```python
from build123d import *

# Parameters (mm, degrees)
SKETCH1_R           = 2.5
BOSS_EXTRUDE1_DEPTH = 370


with BuildPart() as part:
    # Sketch1 → Boss-Extrude1 (new body)
    with BuildSketch(Plane(origin=(0, 0, 0), x_dir=(1, 0, 0), z_dir=(0, 1, 0))):
        with BuildLine():
            Line((-10, 4.65), (-9.8, 4.65))
            Line((-9.8, 4.65), (-9.8, 4.4))
            ThreePointArc((-9.8, 4.4), (-9.741421356, 4.258578644), (-9.6, 4.2))
            Line((-9.6, 4.2), (-8.4, 4.2))
            ThreePointArc((-8.4, 4.2), (-8.258578644, 4.258578644), (-8.2, 4.4))
            Line((-8.2, 4.4), (-8.2, 5.45))
            ThreePointArc((-8.2, 5.45), (-8.141421356, 5.591421356), (-8, 5.65))
            Line((-8, 5.65), (-6.832842712, 5.65))
            ThreePointArc((-6.832842712, 5.65), (-6.756306026, 5.634775907), (-6.691421356, 5.591421356))
            Line((-6.691421356, 5.591421356), (-4.058578644, 2.958578644))
            ThreePointArc((-4.058578644, 2.958578644), (-4.015224093, 2.893693974), (-4, 2.817157288))
            Line((-4, 2.817157288), (-4, -2.817157288))
            ThreePointArc((-4, -2.817157288), (-4.015224093, -2.893693974), (-4.058578644, -2.958578644))
            Line((-4.058578644, -2.958578644), (-6.691421356, -5.591421356))
            ThreePointArc((-6.691421356, -5.591421356), (-6.756306026, -5.634775907), (-6.832842712, -5.65))
            Line((-6.832842712, -5.65), (-8, -5.65))
            ThreePointArc((-8, -5.65), (-8.141421356, -5.591421356), (-8.2, -5.45))
            Line((-8.2, -5.45), (-8.2, -4.4))
            ThreePointArc((-8.2, -4.4), (-8.258578644, -4.258578644), (-8.4, -4.2))
            Line((-8.4, -4.2), (-9.6, -4.2))
            ThreePointArc((-9.6, -4.2), (-9.741421356, -4.258578644), (-9.8, -4.4))
            Line((-9.8, -4.4), (-9.8, -4.65))
            Line((-9.8, -4.65), (-10, -4.65))
            Line((-10, -4.65), (-10, -9.8))
            ThreePointArc((-10, -9.8), (-9.941421356, -9.941421356), (-9.8, -10))
            Line((-9.8, -10), (-4.65, -10))
            Line((-4.65, -10), (-4.65, -9.8))
            Line((-4.65, -9.8), (-4.4, -9.8))
            ThreePointArc((-4.4, -9.8), (-4.258578644, -9.741421356), (-4.2, -9.6))
            Line((-4.2, -9.6), (-4.2, -8.4))
            ThreePointArc((-4.2, -8.4), (-4.258578644, -8.258578644), (-4.4, -8.2))
            Line((-4.4, -8.2), (-5.45, -8.2))
            ThreePointArc((-5.45, -8.2), (-5.591421356, -8.141421356), (-5.65, -8))
            Line((-5.65, -8), (-5.65, -6.832842712))
            ThreePointArc((-5.65, -6.832842712), (-5.634775907, -6.756306026), (-5.591421356, -6.691421356))
            Line((-5.591421356, -6.691421356), (-2.958578644, -4.058578644))
            ThreePointArc((-2.958578644, -4.058578644), (-2.893693974, -4.015224093), (-2.817157288, -4))
            Line((-2.817157288, -4), (2.817157288, -4))
            ThreePointArc((2.817157288, -4), (2.893693974, -4.015224093), (2.958578644, -4.058578644))
            Line((2.958578644, -4.058578644), (5.591421356, -6.691421356))
            ThreePointArc((5.591421356, -6.691421356), (5.634775907, -6.756306026), (5.65, -6.832842712))
            Line((5.65, -6.832842712), (5.65, -8))
            ThreePointArc((5.65, -8), (5.591421356, -8.141421356), (5.45, -8.2))
            Line((5.45, -8.2), (4.4, -8.2))
            ThreePointArc((4.4, -8.2), (4.258578644, -8.258578644), (4.2, -8.4))
            Line((4.2, -8.4), (4.2, -9.6))
            ThreePointArc((4.2, -9.6), (4.258578644, -9.741421356), (4.4, -9.8))
            Line((4.4, -9.8), (4.65, -9.8))
            Line((4.65, -9.8), (4.65, -10))
            Line((4.65, -10), (9.8, -10))
            ThreePointArc((9.8, -10), (9.941421356, -9.941421356), (10, -9.8))
            Line((10, -9.8), (10, -4.65))
            Line((10, -4.65), (9.8, -4.65))
            Line((9.8, -4.65), (9.8, -4.4))
            ThreePointArc((9.8, -4.4), (9.741421356, -4.258578644), (9.6, -4.2))
            Line((9.6, -4.2), (8.4, -4.2))
            ThreePointArc((8.4, -4.2), (8.258578644, -4.258578644), (8.2, -4.4))
            Line((8.2, -4.4), (8.2, -5.45))
            ThreePointArc((8.2, -5.45), (8.141421356, -5.591421356), (8, -5.65))
            Line((8, -5.65), (6.832842712, -5.65))
            ThreePointArc((6.832842712, -5.65), (6.756306026, -5.634775907), (6.691421356, -5.591421356))
            Line((6.691421356, -5.591421356), (4.058578644, -2.958578644))
            ThreePointArc((4.058578644, -2.958578644), (4.015224093, -2.893693974), (4, -2.817157288))
            Line((4, -2.817157288), (4, 2.817157288))
            ThreePointArc((4, 2.817157288), (4.015224093, 2.893693974), (4.058578644, 2.958578644))
            Line((4.058578644, 2.958578644), (6.691421356, 5.591421356))
            ThreePointArc((6.691421356, 5.591421356), (6.756306026, 5.634775907), (6.832842712, 5.65))
            Line((6.832842712, 5.65), (8, 5.65))
            ThreePointArc((8, 5.65), (8.141421356, 5.591421356), (8.2, 5.45))
            Line((8.2, 5.45), (8.2, 4.4))
            ThreePointArc((8.2, 4.4), (8.258578644, 4.258578644), (8.4, 4.2))
            Line((8.4, 4.2), (9.6, 4.2))
            ThreePointArc((9.6, 4.2), (9.741421356, 4.258578644), (9.8, 4.4))
            Line((9.8, 4.4), (9.8, 4.65))
            Line((9.8, 4.65), (10, 4.65))
            Line((10, 4.65), (10, 9.8))
            ThreePointArc((10, 9.8), (9.941421356, 9.941421356), (9.8, 10))
            Line((9.8, 10), (4.65, 10))
            Line((4.65, 10), (4.65, 9.8))
            Line((4.65, 9.8), (4.4, 9.8))
            ThreePointArc((4.4, 9.8), (4.258578644, 9.741421356), (4.2, 9.6))
            Line((4.2, 9.6), (4.2, 8.4))
            ThreePointArc((4.2, 8.4), (4.258578644, 8.258578644), (4.4, 8.2))
            Line((4.4, 8.2), (5.45, 8.2))
            ThreePointArc((5.45, 8.2), (5.591421356, 8.141421356), (5.65, 8))
            Line((5.65, 8), (5.65, 6.832842712))
            ThreePointArc((5.65, 6.832842712), (5.634775907, 6.756306026), (5.591421356, 6.691421356))
            Line((5.591421356, 6.691421356), (2.958578644, 4.058578644))
            ThreePointArc((2.958578644, 4.058578644), (2.893693974, 4.015224093), (2.817157288, 4))
            Line((2.817157288, 4), (-2.817157288, 4))
            ThreePointArc((-2.817157288, 4), (-2.893693974, 4.015224093), (-2.958578644, 4.058578644))
            Line((-2.958578644, 4.058578644), (-5.591421356, 6.691421356))
            ThreePointArc((-5.591421356, 6.691421356), (-5.634775907, 6.756306026), (-5.65, 6.832842712))
            Line((-5.65, 6.832842712), (-5.65, 8))
            ThreePointArc((-5.65, 8), (-5.591421356, 8.141421356), (-5.45, 8.2))
            Line((-5.45, 8.2), (-4.4, 8.2))
            ThreePointArc((-4.4, 8.2), (-4.258578644, 8.258578644), (-4.2, 8.4))
            Line((-4.2, 8.4), (-4.2, 9.6))
            ThreePointArc((-4.2, 9.6), (-4.258578644, 9.741421356), (-4.4, 9.8))
            Line((-4.4, 9.8), (-4.65, 9.8))
            Line((-4.65, 9.8), (-4.65, 10))
            Line((-4.65, 10), (-9.8, 10))
            ThreePointArc((-9.8, 10), (-9.941421356, 9.941421356), (-10, 9.8))
            Line((-10, 9.8), (-10, 4.65))
        make_face()
        Circle(SKETCH1_R, mode=Mode.SUBTRACT)
    extrude(amount=BOSS_EXTRUDE1_DEPTH)


solid = part.part
```
The listing builds one solid part. Answer for the finished solid, in the listing's coordinates (mm). A direction names the side the tool comes from. Round coordinates to 2 decimals unless told otherwise and drop trailing zeros. Use one line per item in the form item = value. Start each with the question number.
1. For a pull along Z with two mould halves and no side action, classify faces 4 (the face through (2, 370, -2)), 5 (the face through (0, 182, 4)), 6 (the face through (-4, 182, 0)) as pulls with the +Z half, pulls with the -Z half, needs draft (parallel to the pull), parting line crosses it, or undercut.
2. A tool of negligible diameter and unlimited length cuts with its end or side. For faces 1 (the face through (4, 182, 0)), 2 (the face through (0, 182, -4)), 3 (the face through (2, 0, -2)), from which of +Z, -Z, +X, -X, +Y, -Y can it reach the whole face along a straight path? Write none if from no direction.
3. Consider line 1 (X direction, y = 316, z = -6.75); line 2 (Z direction, x = 9, y = 283.5); line 3 (X direction, y = 225, z = 0). Determine where each line is inside the solid, lowest interval first. Write a range as [from, to].
4. Given pin 1 Ø1.5 at (y, z) = (298, -2) entering from +X; pin 2 Ø1.5 at (x, z) = (-1, -6) entering from -Y; pin 3 Ø8 at (x, y) = (4.5, 42.5) entering from +Z; pin 4 Ø6 at (y, z) = (122.5, -1.5) entering from -X, each flat-ended and moving along its own axis, determine where each tip first touches the part or whether it passes through.
Geometry check:
q1.face_4 = needs draft
q1.face_5 = pulls with the +Z half
q1.face_6 = undercut
q2.face_1 = +X, +Y, -Y
q2.face_2 = -Z, +Y, -Y
q2.face_3 = +Z, -Z, +X, -X, -Y
q3.line_1 = [-10, -5.63], [5.63, 10]
q3.line_2 = [-10, -4.2], [4.2, 10]
q3.line_3 = [-4, -2.5], [2.5, 4]
q4.pin_1 = 4
q4.pin_2 = through
q4.pin_3 = 10
q4.pin_4 = -9.8
